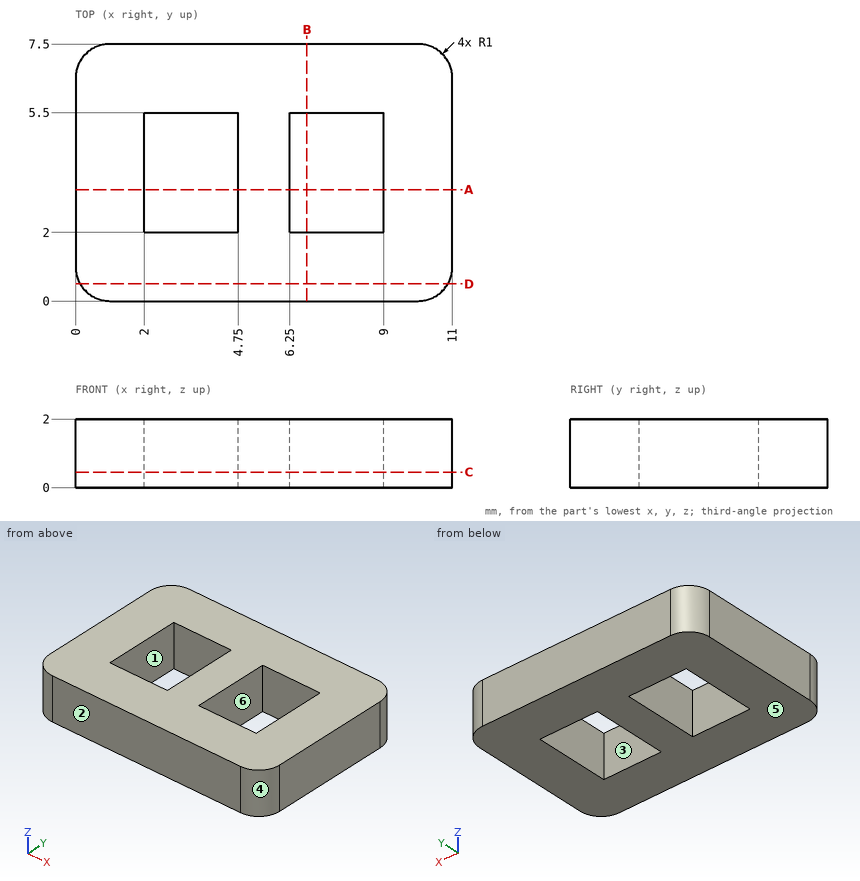
Geometry check sheet. Reference: drawing and pictorial views, mm from the part's lowest x, y, z. A direction names the side the tool comes from. Round coordinates to 2 decimals unless told otherwise and drop trailing zeros. Write each loop counter-clockwise with the first axis right and the second up, starting at its lowest first coordinate (ties: lowest second). Pieces come first, ordered by that corner, then holes. Notation, with made-up numbers: (24.25, 74.25) -> (30.25, 74.25) arc R12 ccw to (30.25, 94.25) -> close; hole circle Ø6 at (24.25, -18). An arc over 180 degrees is marked (long way). Put each result on its own line as item: value.
1) Access from +Z, -Z, +X, -X, +Y, -Y to the whole of each face (thin tool, end or side, straight path). Record for the marked faces 1 and 2.
Recorded:
face 1: +Z, -Z
face 2: +Z, -Z, +X, -X, -Y
2) Thickness scan on probe 1 along X at (y, z) = (4, 0.1); probe 2 along Y at (x, z) = (8, 1.15); probe 3 along Y at (x, z) = (10.5, 1.15). Record the ranges inside material, lowest first. Write a range as from..to.
Recorded:
probe 1: x = 0..2, 4.75..6.25, 9..11
probe 2: y = 0..2, 5.5..7.5
probe 3: y = 0.13..7.37
3) Cross-section at A-A, the plane y = 3.25. Enter the section's corners in (x, z), plus the area to 3 significant figures.
Recorded:
outline: (0, 0) -> (2, 0) -> (2, 2) -> (0, 2) -> close; (4.75, 0) -> (6.25, 0) -> (6.25, 2) -> (4.75, 2) -> close; (9, 0) -> (11, 0) -> (11, 2) -> (9, 2) -> close
area: 11.0 mm2
4) Cross-section at C-C, the plane z = 0.45. Enter the section's corners in (x, y), plus the area to 3 significant figures.
Recorded:
outline: (0, 1) arc R1 ccw to (1, 0) -> (10, 0) arc R1 ccw to (11, 1) -> (11, 6.5) arc R1 ccw to (10, 7.5) -> (1, 7.5) arc R1 ccw to (0, 6.5) -> close; hole (2, 2) -> (4.75, 2) -> (4.75, 5.5) -> (2, 5.5) -> close; hole (6.25, 2) -> (9, 2) -> (9, 5.5) -> (6.25, 5.5) -> close
area: 62.4 mm2
5) Release check for a two-part mould opening along X. For the marked faces 3, 4, 5 and 6 record: pulls with the +X half, pulls with the -X half, needs draft (parallel to the pull), parting line crosses it, or undercut.
Recorded:
face 3: undercut
face 4: pulls with the +X half
face 5: needs draft
face 6: undercut
6) Cross-section at B-B, the plane x = 6.75. Enter the section's corners in (y, z).
Recorded:
outline: (0, 0) -> (2, 0) -> (2, 2) -> (0, 2) -> close; (5.5, 0) -> (7.5, 0) -> (7.5, 2) -> (5.5, 2) -> close
7) Cross-section at D-D, the plane y = 0.5. Enter the section's corners in (x, z), plus the area to 3 significant figures.
Recorded:
outline: (0.13, 0) -> (10.87, 0) -> (10.87, 2) -> (0.13, 2) -> close
area: 21.5 mm2
